Autodesk Inventor part; units mm, degrees
ref_plane "YZ Plane" through (0, 0, 0) normal (1, 0, 0) x (0, 1, 0)
ref_plane "XZ Plane" through (0, 0, 0) normal (0, 1, 0) x (-1, 0, 0)
ref_plane "XY Plane" through (0, 0, 0) normal (0, 0, 1) x (1, 0, 0)
sketch "Sketch1" plane through (0, 0, 0) normal (0, 1, 0) x (-1, 0, 0)
  line L0 (-5, 44.25) -> (5, 44.25)
  line L1 (5, 44.25) -> (5, -44.25)
  line L2 (5, -44.25) -> (-5, -44.25)
  line L3 (-5, -44.25) -> (-5, 44.25)
  line L4 (-5, 44.25) -> (5, -44.25) construction
  line L5 (5, 44.25) -> (-5, -44.25) construction
  point P0 (0, 0)
  dimension "d0" = 88.5
  dimension "d1" = 10
extrude "Extrusion1" add sketch "Sketch1" along normal blind 11
sketch "Sketch2" plane through (-5, 0, 44.25) normal (0, 0, 1) x (1, 0, 0)
  line L0 (10, 0) -> (0, 0)
  line L1 (5, 0) -> (0, 0)
  line L2 (0, 0) -> (0, 4)
  line L3 (0, 4) -> (2.5, 4)
  line L4 (2.5, 4) -> (2.5, 8)
  line L5 (2.5, 8) -> (0, 8)
  line L6 (0, 8) -> (0, 11)
  line L7 (0, 11) -> (5, 11)
  line L8 (0, 11) -> (10, 11)
  line L9 (5, 11) -> (5, 0) construction
  line L10 (0, 0) -> (10, 0)
  line L11 (10, 0) -> (10, 4)
  line L12 (10, 4) -> (7.5, 4)
  line L13 (7.5, 4) -> (7.5, 8)
  line L14 (7.5, 8) -> (10, 8)
  line L15 (10, 8) -> (10, 11)
  line L16 (10, 11) -> (5, 11)
  dimension "d4" = 3
  dimension "d5" = 4
  dimension "d6" = 2.5
extrude "Extrusion2" cut sketch "Sketch2" against normal through all keep common part
sketch "Sketch3" plane through (0, 0, 0) normal (0, -1, 0) x (1, 0, 0)
  line L0 (0, 0) -> (0, 39.25) construction
  circle A0 centre (0, 39.25) radius 1.25
  line L1 (5, -44.25) -> (5, 44.25) construction
  line L2 (5, 0) -> (-5, 0) construction
  line L3 (-5, 44.25) -> (-5, -44.25) construction
  circle A1 centre (0, -39.25) radius 1.25
  dimension "d9" = 2.5
  dimension "d10" = 39.25
extrude "Extrusion3" cut sketch "Sketch3" against normal blind 4
sketch "Sketch4" plane through (0, 11, 0) normal (0, 1, 0) x (1, 0, 0)
  line L0 (-2, 11) -> (2, 11)
  line L1 (2, 11) -> (2, -9)
  line L2 (2, -9) -> (-2, -9)
  line L3 (-2, -9) -> (-2, 11)
  line L4 (-2, 11) -> (2, -9) construction
  line L5 (2, 11) -> (-2, -9) construction
  line L6 (0, 1) -> (0, 0) construction
  dimension "d13" = 4
  dimension "d14" = 20
  dimension "d15" = 1
extrude "Extrusion4" cut sketch "Sketch4" against normal through all
sketch "Sketch5" plane through (0, 11, 0) normal (0, 1, 0) x (1, 0, 0)
  line L0 (-2, -9) -> (-2, 11)
  line L1 (-2, 11) -> (2, 11)
  line L2 (2, 11) -> (2, -9)
  line L3 (-1.5, -9) -> (-1.5, 10.5)
  line L4 (-1.5, 10.5) -> (1.5, 10.5)
  line L5 (1.5, 10.5) -> (1.5, -9)
  line L6 (-1.5, -9) -> (1.5, -9)
  line L7 (2, -9) -> (-2, -9)
  point P0 (0, 0)
  dimension "d18" = 0.5
extrude "Extrusion5" add sketch "Sketch5" against normal blind 1 contours L3 L4 L5 L6
fillet "Fillet1" radius 4 1 edges at (0, 10, 9)
sketch "Sketch7" plane through (0, 11, 0) normal (0, 1, 0) x (1, 0, 0)
  line L0 (1.5, 10.5) -> (-1.5, 10.5) construction
  line L1 (-1.5, 10.5) -> (1.5, 10.5) construction
  line L2 (1.5, 10.5) -> (1.5, 7.5) construction
  line L3 (1.5, 7.5) -> (-1.5, 7.5) construction
  line L4 (-1.5, 7.5) -> (-1.5, 10.5) construction
  line L5 (1.5, -9) -> (1.5, 10.5)
  line L6 (-1.5, 10.5) -> (1.5, 7.5) construction
  circle A0 centre (0, 9) radius 1.5
  line L7 (0, 9) -> (1.5, 9)
  line L8 (0, 9) -> (-1.5, 9)
  point P0 (0, 0)
  dimension "d24" = 3
  dimension "d25" = 3
revolve "Revolution1" add sketch "Sketch7" angle 180 about axis through (0, 11, -9) along (1, 0, 0) picked at (0.9282, 9.352) contours L7 L8 A0
properties part number "Screen Docking rail"
Verification items for the finished model (mm, model axes). A direction names the side the tool comes from. Coordinates: 2 decimals unless noted, no trailing zeros. Loops run counter-clockwise (first coordinate to the right, second up) from the corner with the lowest first, then second, coordinate; pieces in that order, holes last. Notation, with made-up numbers: (70, 18.25) -> (91, 18.25) arc R24 ccw to (91, 46.25) -> close; hole circle Ø4 at (3, -5). An arc over 180 degrees is marked (long way). Answer in a Markdown table with one row per item. Add a question column.
1. Access from +Z, -Z, +X, -X, +Y, -Y to the whole of each face (thin tool, end or side, straight path). Record for faces 5 (the face through (-4, 8, 1)), 6 (the face through (2.5, 6, 1)), 7 (the face through (-1.2, 11, -10.2)).
2. Material ranges on probe 1 along Z at (x, y) = (0, 1.1); probe 2 along Y at (x, z) = (3.5, -2); probe 3 along Z at (x, y) = (0.75, 10.75), recorded low to high. Write a range as [from, to].
3. Section check A-A, the plane z = 0. Enter the section's corners in (x, y).
4. Draft check along X on faces 1 (the face through (4, 8, 1)), 2 (the face through (-2.5, 6, 1)), 3 (the face through (-2, 6, -1)), 4 (the face through (0, 6, -11)). Enter one of: +X half, -X half, draft (parallel to the pull), parting line (faces both ways), or undercut.
5. Section check D-D, the plane z = 26.5. Enter the section's corners in (x, y).
6. Depth check by flat-ended pin: P1, Ø0.9, axis at x = 0.5, z = -4, coming from the -Y side; P2, Ø3, axis at x = 1.5, z = -19, coming from the +Y side; P3, Ø1.6, axis at x = -0.5, z = -10, coming from the +Y side. Enter the tip coordinate at first touch or a pass-through.
7. Section check B-B, the plane y = 2.5. Enter the section's corners in (x, z), then the cut area to 3 significant figures.
8. Section check C-C, the plane z = -39.25. Enter the section's corners in (x, y), then the cut area to 3 significant figures.
Derived:
| question | item | result |
|---|---|---|
| 1 | face 5 | +Z, -Z, -X |
| 1 | face 6 | +Z, -Z, +X |
| 1 | face 7 | -Z, -X, +Y |
| 2 | probe 1 | z = [-44.25, -40.5], [-38, -11], [9, 38], [40.5, 44.25] |
| 2 | probe 2 | y = [0, 4], [8, 11] |
| 2 | probe 3 | z = [-44.25, -11], [-10.5, 44.25] |
| 3 | outline | (-5, 0) -> (-2, 0) -> (-2, 11) -> (-5, 11) -> (-5, 8) -> (-2.5, 8) -> (-2.5, 4) -> (-5, 4) -> close; (-1.5, 10) -> (1.5, 10) -> (1.5, 11) -> (-1.5, 11) -> close; (2, 0) -> (5, 0) -> (5, 4) -> (2.5, 4) -> (2.5, 8) -> (5, 8) -> (5, 11) -> (2, 11) -> close |
| 4 | face 1 | draft |
| 4 | face 2 | -X half |
| 4 | face 3 | undercut |
| 4 | face 4 | undercut |
| 5 | outline | (-5, 0) -> (5, 0) -> (5, 4) -> (2.5, 4) -> (2.5, 8) -> (5, 8) -> (5, 11) -> (-5, 11) -> (-5, 8) -> (-2.5, 8) -> (-2.5, 4) -> (-5, 4) -> close |
| 6 | P1 | stops at y = 10 |
| 6 | P2 | stops at y = 11 |
| 6 | P3 | stops at y = 12.47 |
| 7 | outline | (-5, -44.25) -> (5, -44.25) -> (5, 44.25) -> (-5, 44.25) -> close; hole (-2, -11) -> (2, -11) -> (2, 9) -> (-2, 9) -> close; hole circle Ø2.5 at (0, -39.25); hole circle Ø2.5 at (0, 39.25) |
| 7 | area | 795 mm² |
| 8 | outline | (-5, 0) -> (-1.25, 0) -> (-1.25, 4) -> (1.25, 4) -> (1.25, 0) -> (5, 0) -> (5, 4) -> (2.5, 4) -> (2.5, 8) -> (5, 8) -> (5, 11) -> (-5, 11) -> (-5, 8) -> (-2.5, 8) -> (-2.5, 4) -> (-5, 4) -> close |
| 8 | area | 80.0 mm² |
